Here's how the part is built. I have some questions about the finished solid (model axes, mm). Face numbers are marked on the shaded views. A direction names the side the tool comes from. Coordinates: 2 decimals unless noted, no trailing zeros. Loops run counter-clockwise (first coordinate to the right, second up) from the corner with the lowest first, then second, coordinate; pieces in that order, holes last. Notation, with made-up numbers: (-25.75, -4.75) -> (28.25, -4.75) arc R6 ccw to (28.25, 3.25) -> close; hole circle Ø11 at (-5, 72). An arc over 180 degrees is marked (long way). Answer as a JSON object with one key per item and string values. Group by question number.
1) I need wall thicknesses on probe 1 along X at (y, z) = (14.25, 25); probe 2 along X at (y, z) = (14.5, 20.5); probe 3 along X at (y, z) = (20.25, -24). Which ranges of each line are inside material? Lowest first, please. Write a range as [from, to].
2) I want a section at C-C (x = -7). Write out the boundary of the cut face in (y, z).
3) I want a section at B-B (z = -12.5). Write out the boundary of the cut face in (x, y), then the cut area to 3 significant figures.
4) Which directions (+Z, -Z, +X, -X, +Y, -Y) give clear straight access to the entire face, cutting with the end or side of a thin tool? Please do the marked faces 1 and 2.
5) If we mould it in two halves opening along X, with no side actions, what happens to the marked faces 3, 4 and 5? For each: +X half, -X half, draft (parallel to the pull), parting line (faces both ways), or undercut.
6) I'm going to push flat-ended pins straight in: pin 1 (11.5 mm diameter, centred on x = 1, z = 4.5, fed in from +Y); pin 2 (2.5 mm diameter, centred on x = -17, z = -25.5, fed in from +Y); pin 3 (1.5 mm diameter, centred on x = 3.5, y = 18, fed in from -Z); pin 4 (3 mm diameter, centred on x = 0, z = 12, fed in from +Y). Where does each tip first touch, or does it pass through?
7) I want a section at A-A (y = 16.5). Count the separate pieces of the cut face and the enclosed holes in it, then the cut area to 3 significant figures.
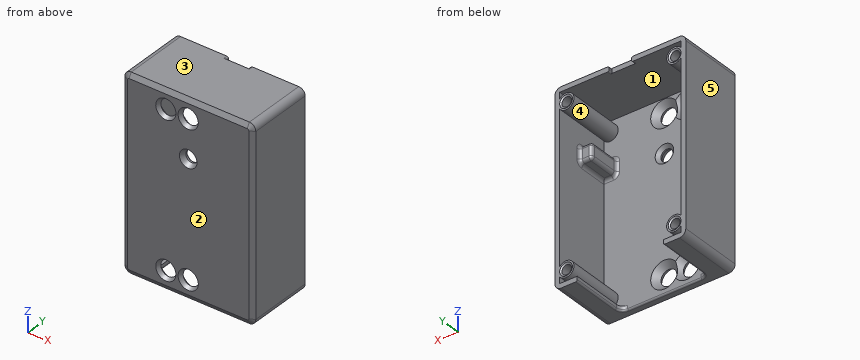
```python
from build123d import *
from OCP.BRepFilletAPI import BRepFilletAPI_MakeChamfer

# Parameters (mm, degrees)
SKETCH_1_W          = 41
SKETCH_1_H          = 60
SKETCH_1_R          = 2.3
SKETCH_1_R_2        = 1.9
EXTRUDE_1_DEPTH     = 3
CHAMFER_1_SIZE      = 2
SKETCH_2_W          = 41
SKETCH_2_H          = 60
SKETCH_2_W_2        = 38
SKETCH_2_H_2        = 57
EXTRUDE_1_2_DEPTH   = 18
SKETCH_3_W          = 27
SKETCH_3_H          = 3.030341357
CUT_EXTRUDE_1_DEPTH = 18
SKETCH_4_R          = 2.5
EXTRUDE_2_DEPTH     = 18
SKETCH_5_R          = 1.5
CUT_EXTRUDE_2_DEPTH = 10
SKETCH_7_W          = 7
SKETCH_7_H          = 4.356080651
CUT_EXTRUDE_3_DEPTH = 1.2
FILLET_2_R          = 0.5
FILLET_3_R          = 2
CHAMFER_4_SIZE      = 0.866025404
CHAMFER_4_SIZE_2    = 1.5
CHAMFER_6_SIZE      = 0.5
CHAMFER_6_SIZE2     = 0.288675135
SKETCH_8_W          = 4
SKETCH_8_H          = 5
EXTRUDE_3_DEPTH     = 10
FILLET_6_R          = 1
FILLET_7_R          = 2
FILLET_8_R          = 0.5
CHAMFER_7_SIZE      = 1


with BuildPart() as part:
    # Эскиз1 → Extrude 1 (new body)
    with BuildSketch(Plane(origin=(0, 0, 0), x_dir=(1, 0, 0), z_dir=(0, 1, 0))):
        Rectangle(SKETCH_1_W, SKETCH_1_H)
        with Locations(Location((0, 24, 0), (0, 0, 270))):
            Circle(SKETCH_1_R, mode=Mode.SUBTRACT)
        with Locations(Location((0, -24, 0), (0, 0, 270))):
            Circle(SKETCH_1_R, mode=Mode.SUBTRACT)
        with Locations(Location((0, -12, 0), (0, 0, 270))):
            Circle(SKETCH_1_R_2, mode=Mode.SUBTRACT)
        with Locations(Location((-7, -24, 0), (0, 0, 90))):
            Circle(SKETCH_1_R, mode=Mode.SUBTRACT)
        with Locations(Location((-7, 24, 0), (0, 0, 90))):
            Circle(SKETCH_1_R, mode=Mode.SUBTRACT)
    extrude(amount=EXTRUDE_1_DEPTH)

    # Фаска1
    # the kernel refuses this chamfer: 2 mm, written as the material it takes off along each edge
    with BuildSketch(Plane(origin=(0, 3, -24), x_dir=(0, 0, 1), z_dir=(-1, 0, 0))) as chamfer_1_piece_1:
        Polygon((2.3, -CHAMFER_1_SIZE), (2.3 + CHAMFER_1_SIZE, 0), (2.3, 0), align=None)
    revolve(axis=Axis((0, 3, -24), (0, 1, 0)), mode=Mode.SUBTRACT)
    with BuildSketch(Plane(origin=(0, 3, 24), x_dir=(0, 0, 1), z_dir=(-1, 0, 0))) as chamfer_1_piece_2:
        Polygon((2.3, -CHAMFER_1_SIZE), (2.3 + CHAMFER_1_SIZE, 0), (2.3, 0), align=None)
    revolve(axis=Axis((0, 3, 24), (0, 1, 0)), mode=Mode.SUBTRACT)
    with BuildSketch(Plane(origin=(-7, 3, 24), x_dir=(0, 0, -1), z_dir=(1, 0, 0))) as chamfer_1_piece_3:
        Polygon((2.3, -CHAMFER_1_SIZE), (2.3 + CHAMFER_1_SIZE, 0), (2.3, 0), align=None)
    revolve(axis=Axis((-7, 3, 24), (0, 1, 0)), mode=Mode.SUBTRACT)
    with BuildSketch(Plane(origin=(-7, 3, -24), x_dir=(0, 0, -1), z_dir=(1, 0, 0))) as chamfer_1_piece_4:
        Polygon((2.3, -CHAMFER_1_SIZE), (2.3 + CHAMFER_1_SIZE, 0), (2.3, 0), align=None)
    revolve(axis=Axis((-7, 3, -24), (0, 1, 0)), mode=Mode.SUBTRACT)

    # Эскиз2 → Extrude 1 2 (add)
    with BuildSketch(Plane(origin=(0, 3, 0), x_dir=(1, 0, 0), z_dir=(0, 1, 0))):
        Rectangle(SKETCH_2_W, SKETCH_2_H)
        Rectangle(SKETCH_2_W_2, SKETCH_2_H_2, mode=Mode.SUBTRACT)
    extrude(amount=EXTRUDE_1_2_DEPTH)

    # Эскиз3 → Вырез-Вытянуть1 (cut)
    with BuildSketch(Plane(origin=(0, 21, 0), x_dir=(1, 0, 0), z_dir=(0, 1, 0))):
        with Locations((0, 29.478101209)):
            Rectangle(SKETCH_3_W, SKETCH_3_H)
    extrude(amount=-CUT_EXTRUDE_1_DEPTH, mode=Mode.SUBTRACT)

    # Эскиз4 → Бобышка-Вытянуть2 (add)
    with BuildSketch(Plane(origin=(0, 3, 0), x_dir=(1, 0, 0), z_dir=(0, 1, 0))):
        with Locations((17, 25)):
            Circle(SKETCH_4_R)
        with Locations((-17, 25)):
            Circle(SKETCH_4_R)
        with Locations((17, -25)):
            Circle(SKETCH_4_R)
        with Locations((-17, -25)):
            Circle(SKETCH_4_R)
    extrude(amount=EXTRUDE_2_DEPTH)

    # Эскиз5 → Вырез-Вытянуть2 (cut)
    with BuildSketch(Plane(origin=(0, 21, 0), x_dir=(1, 0, 0), z_dir=(0, 1, 0))):
        with Locations(Location((17, 25, 0), (0, 0, 270))):
            Circle(SKETCH_5_R)
        with Locations(Location((17, -25, 0), (0, 0, 270))):
            Circle(SKETCH_5_R)
        with Locations(Location((-17, -25, 0), (0, 0, 270))):
            Circle(SKETCH_5_R)
        with Locations(Location((-17, 25, 0), (0, 0, 270))):
            Circle(SKETCH_5_R)
    extrude(amount=-CUT_EXTRUDE_2_DEPTH, mode=Mode.SUBTRACT)

    # Эскиз7 → Вырез-Вытянуть3 (cut)
    with BuildSketch(Plane(origin=(0, 21, 0), x_dir=(1, 0, 0), z_dir=(0, 1, 0))):
        with Locations((0, -28.804800006)):
            Rectangle(SKETCH_7_W, SKETCH_7_H)
    extrude(amount=-CUT_EXTRUDE_3_DEPTH, mode=Mode.SUBTRACT)

    # Скругление2
    fillet_2_edges = [part.edges().sort_by_distance(p)[0] for p in [
        (-3.5, 20.4, 28.5),
        (3.5, 20.4, 28.5),
        (3.5, 20.4, 30),
        (-3.5, 20.4, 30),
    ]]
    fillet(fillet_2_edges, radius=FILLET_2_R)

    # Скругление3
    fillet_3_edges = [part.edges().sort_by_distance(p)[0] for p in [
        (20.5, 10.5, 30),
        (-20.5, 10.5, 30),
        (-20.5, 10.5, -30),
        (20.5, 10.5, -30),
    ]]
    fillet(fillet_3_edges, radius=FILLET_3_R)

    # Фаска4
    # the kernel refuses this chamfer: 1.5, 0.866025404 mm, written as the material it takes off along each edge
    with BuildSketch(Plane(origin=(0, 0, 24), x_dir=(0, 0, 1), z_dir=(-1, 0, 0))) as chamfer_4_piece_1:
        Polygon((2.3 + CHAMFER_4_SIZE, 0), (2.3, CHAMFER_4_SIZE_2), (2.3, 0), align=None)
    revolve(axis=Axis((0, 0, 24), (0, 1, 0)), mode=Mode.SUBTRACT)
    with BuildSketch(Plane(origin=(18.5, 0, -30), x_dir=(0, -0.01932676561270073, 0.999813220622208), z_dir=(-1, 0, 0))) as chamfer_4_piece_2:
        Polygon((CHAMFER_4_SIZE_2 * 0.999813220622, CHAMFER_4_SIZE_2 * 0.0193267656127), (-CHAMFER_4_SIZE * 0.0193267656079, CHAMFER_4_SIZE * 0.999813220373), (0, 0), align=None)
    extrude(amount=37, mode=Mode.SUBTRACT)
    with BuildSketch(Plane(origin=(-20.5, 0, -28), x_dir=(0.999813220622208, -0.01932676561270073, 0), z_dir=(0, 0, 1)), Plane(origin=(20.5, 0, 28), x_dir=(-0.999813220622208, -0.01932676561270073, 0), z_dir=(0, 0, -1))) as chamfer_4_piece_3:
        Polygon((CHAMFER_4_SIZE_2 * 0.999813220622, CHAMFER_4_SIZE_2 * 0.0193267656127), (-CHAMFER_4_SIZE * 0.0193267656079, CHAMFER_4_SIZE * 0.999813220373), (0, 0), align=None)
    extrude(amount=56, mode=Mode.SUBTRACT)
    with BuildSketch(Plane(origin=(-18.5, 0, 30), x_dir=(0, 0.9983227437537924, 0.0578938624026721), z_dir=(1, 0, 0))) as chamfer_4_piece_4:
        Polygon((CHAMFER_4_SIZE * 0.998322743505, -CHAMFER_4_SIZE * 0.0578938623883), (-CHAMFER_4_SIZE_2 * 0.0578938624027, -CHAMFER_4_SIZE_2 * 0.998322743754), (0, 0), align=None)
    extrude(amount=37, mode=Mode.SUBTRACT)
    with BuildSketch(Plane(origin=(-18.5, 0, -28), x_dir=(0, 0, -1), z_dir=(1, 0, 0))) as chamfer_4_piece_5:
        Polygon((2 - CHAMFER_4_SIZE_2, 0), (2, CHAMFER_4_SIZE), (2, 0), align=None)
    revolve(axis=Axis((-18.5, 0, -28), (0, 1, 0)), revolution_arc=90, mode=Mode.SUBTRACT)
    with BuildSketch(Plane(origin=(-18.5, 0, 28), x_dir=(0, 0, 1), z_dir=(1, 0, 0))) as chamfer_4_piece_6:
        Polygon((2 - CHAMFER_4_SIZE_2, 0), (2, -CHAMFER_4_SIZE), (2, 0), align=None)
    revolve(axis=Axis((-18.5, 0, 28), (0, -1, 0)), revolution_arc=90, mode=Mode.SUBTRACT)
    with BuildSketch(Plane(origin=(18.5, 0, 28), x_dir=(0, 0, 1), z_dir=(-1, 0, 0))) as chamfer_4_piece_7:
        Polygon((2, CHAMFER_4_SIZE), (2 - CHAMFER_4_SIZE_2, 0), (2, 0), align=None)
    revolve(axis=Axis((18.5, 0, 28), (0, 1, 0)), revolution_arc=90, mode=Mode.SUBTRACT)
    with BuildSketch(Plane(origin=(18.5, 0, -28), x_dir=(0, 0, -1), z_dir=(-1, 0, 0))) as chamfer_4_piece_8:
        Polygon((2 - CHAMFER_4_SIZE_2, 0), (2, -CHAMFER_4_SIZE), (2, 0), align=None)
    revolve(axis=Axis((18.5, 0, -28), (0, -1, 0)), revolution_arc=90, mode=Mode.SUBTRACT)
    with BuildSketch(Plane(origin=(0, 0, -24), x_dir=(0, 0, 1), z_dir=(-1, 0, 0))) as chamfer_4_piece_9:
        Polygon((2.3 + CHAMFER_4_SIZE, 0), (2.3, CHAMFER_4_SIZE_2), (2.3, 0), align=None)
    revolve(axis=Axis((0, 0, -24), (0, 1, 0)), mode=Mode.SUBTRACT)
    with BuildSketch(Plane(origin=(0, 0, 12), x_dir=(0, 0, 1), z_dir=(-1, 0, 0))) as chamfer_4_piece_10:
        Polygon((1.9 + CHAMFER_4_SIZE, 0), (1.9, CHAMFER_4_SIZE_2), (1.9, 0), align=None)
    revolve(axis=Axis((0, 0, 12), (0, 1, 0)), mode=Mode.SUBTRACT)
    with BuildSketch(Plane(origin=(-7, 0, -24), x_dir=(0, 0, -1), z_dir=(1, 0, 0))) as chamfer_4_piece_11:
        Polygon((2.3 + CHAMFER_4_SIZE, 0), (2.3, CHAMFER_4_SIZE_2), (2.3, 0), align=None)
    revolve(axis=Axis((-7, 0, -24), (0, 1, 0)), mode=Mode.SUBTRACT)
    with BuildSketch(Plane(origin=(-7, 0, 24), x_dir=(0, 0, -1), z_dir=(1, 0, 0))) as chamfer_4_piece_12:
        Polygon((2.3 + CHAMFER_4_SIZE, 0), (2.3, CHAMFER_4_SIZE_2), (2.3, 0), align=None)
    revolve(axis=Axis((-7, 0, 24), (0, 1, 0)), mode=Mode.SUBTRACT)

    # Фаска6: one chamfer whose edges measure the first distance from different faces: ONE call of the kernel's chamfer builder (chamfer() names one face for all edges)
    chamfer_6_edges_1 = [part.edges().sort_by_distance(p)[0] for p in [
        (-17, 21, -26.5),
        (-17, 21, 23.5),
    ]]
    chamfer_6_side_1 = [part.faces().sort_by_distance(p)[0] for p in [
        (-11.25, 21, 29.376381527),
    ]]
    chamfer_6_edges_2 = [part.edges().sort_by_distance(p)[0] for p in [
        (17, 21, 23.5),
        (17, 21, -26.5),
    ]]
    chamfer_6_side_2 = [part.faces().sort_by_distance(p)[0] for p in [
        (11.25, 21, 29.376381527),
    ]]
    chamfer_6 = BRepFilletAPI_MakeChamfer(part.part.solid().wrapped)
    for e in chamfer_6_edges_1:
        chamfer_6.Add(CHAMFER_6_SIZE, CHAMFER_6_SIZE2, e.wrapped, chamfer_6_side_1[0].wrapped)  # the first distance lies on this face
    for e in chamfer_6_edges_2:
        chamfer_6.Add(CHAMFER_6_SIZE, CHAMFER_6_SIZE2, e.wrapped, chamfer_6_side_2[0].wrapped)  # the first distance lies on this face
    add(Compound.cast(chamfer_6.Shape()), mode=Mode.REPLACE)

    # Эскиз8 → Бобышка-Вытянуть3 (add)
    with BuildSketch(Plane(origin=(0, 3, 0), x_dir=(1, 0, 0), z_dir=(0, 1, 0))):
        with Locations((17, -14)):
            Rectangle(SKETCH_8_W, SKETCH_8_H)
        with Locations((-17, -5.5)):
            Rectangle(SKETCH_8_W, SKETCH_8_H)
    extrude(amount=EXTRUDE_3_DEPTH)

    # Скругление6
    fillet_6_edges = [part.edges().sort_by_distance(p)[0] for p in [
        (19, 8, 16.5),
        (17, 3, 11.5),
        (19, 8, 11.5),
        (15, 3, 14),
        (15, 8, 11.5),
        (17, 3, 16.5),
        (15, 8, 16.5),
        (19, 13, 14),
        (17, 13, 11.5),
        (15, 13, 14),
        (17, 13, 16.5),
        (-19, 8, 3),
        (-17, 3, 8),
        (-19, 8, 8),
        (-15, 3, 5.5),
        (-15, 8, 8),
        (-17, 3, 3),
        (-15, 8, 3),
        (-19, 13, 5.5),
        (-17, 13, 8),
        (-15, 13, 5.5),
        (-17, 13, 3),
    ]]
    fillet(fillet_6_edges, radius=FILLET_6_R)

    # Скругление7
    fillet_7_edges = [part.edges().sort_by_distance(p)[0] for p in [
        (-13.5, 3, -29.25),
        (13.5, 3, -29.25),
    ]]
    fillet(fillet_7_edges, radius=FILLET_7_R)

    # Скругление8
    fillet_8_edges = [part.edges().sort_by_distance(p)[0] for p in [
        (0, 3, -30),
        (13.5, 13, -30),
        (12.914213562, 3.585786438, -30),
        (-12.914213562, 3.585786438, -30),
        (-13.5, 13, -30),
    ]]
    fillet(fillet_8_edges, radius=FILLET_8_R)

    # Фаска7
    chamfer_7_edges = [part.edges().sort_by_distance(p)[0] for p in [
        (0, 3, 10.1),
    ]]
    chamfer(chamfer_7_edges, length=CHAMFER_7_SIZE)


solid = part.part
```
Determined:
{
 "1": {"probe 1": "[-20.5, -18.5], [-15.5, -14.5], [14.5, 15.5], [18.5, 20.5]", "probe 2": "[-20.5, -19], [19, 20.5]", "probe 3": "[-20.5, -18.12], [-15.88, -14.71], [14.71, 15.88], [18.12, 20.5]"},
 "2": {"outline": "(0, -28.5) -> (0.87, -30) -> (2.5, -30) arc R0.5 ccw to (3, -29.5) -> (3, -28.3) -> (1.18, -26.48) -> (0, -27.17) -> close; (0, -20.83) -> (1.18, -21.52) -> (3, -19.7) -> (3, 19.7) -> (1.18, 21.52) -> (0, 20.83) -> close; (0, 27.17) -> (1.18, 26.48) -> (3, 28.3) -> (3, 28.5) -> (21, 28.5) -> (21, 30) -> (0.87, 30) -> (0, 28.5) -> close"},
 "3": {"outline": "(-20.5, 0.87) -> (-19, 0) -> (19, 0) -> (20.5, 0.87) -> (20.5, 21) -> (19, 21) -> (19, 3) -> (-19, 3) -> (-19, 21) -> (-20.5, 21) -> close", "area": "176 mm^2"},
 "4": {"face 1": "+Y", "face 2": "+Z, -Z, +X, -X, -Y"},
 "5": {"face 3": "draft", "face 4": "undercut", "face 5": "-X half"},
 "6": {"pin 1": "y = 3", "pin 2": "y = 20.86", "pin 3": "z = 28.5", "pin 4": "through"},
 "7": {"separate pieces": "1", "enclosed holes": "4", "area": "296 mm^2"}
}
